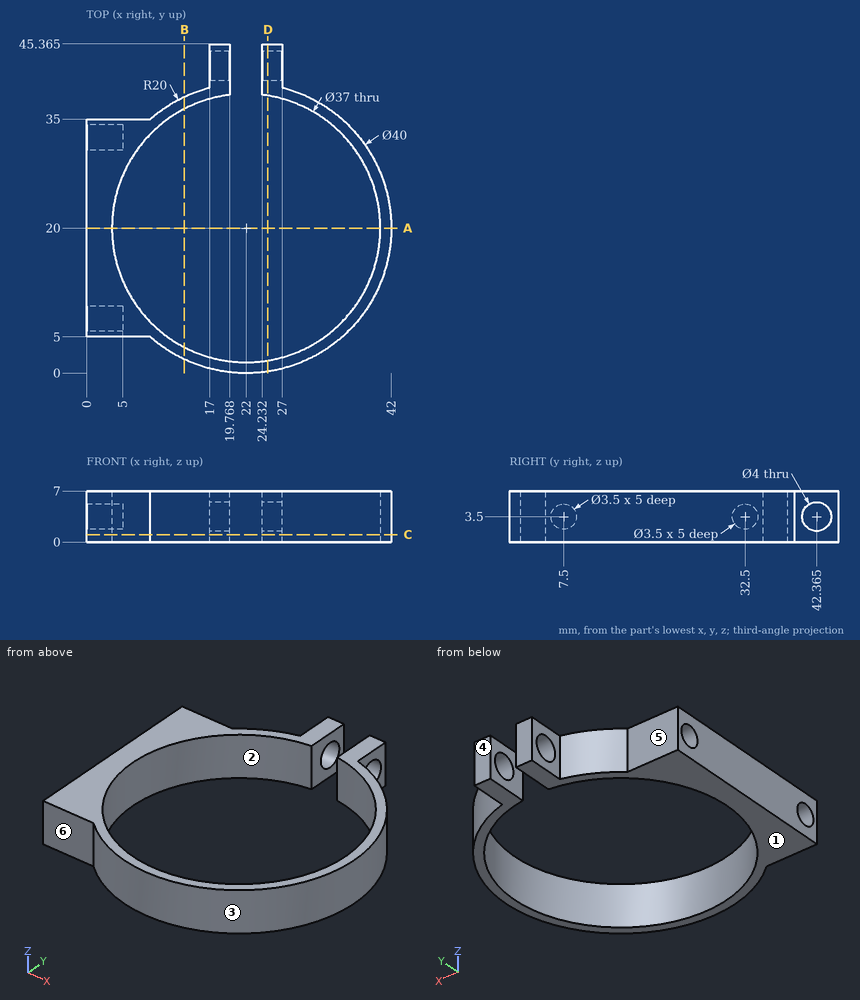
Geometry check sheet. Reference: drawing and pictorial views, mm from the part's lowest x, y, z. A direction names the side the tool comes from. Coordinates: 2 decimals unless noted, no trailing zeros. Order: outer loops, then holes, each group sorted by start corner. A loop starts at its lowest first (then second) coordinate and runs counter-clockwise, first axis right, second up.
Item 1: Mould release check, pull along X, two halves, no side actions. Record for the marked faces 1, 2 and 3: released by +X, released by -X, zero draft, split by the parting line, or undercut.
Item 2: Scan lines: line 1 along Y through (x, z) = (2, 3.5); line 2 along Y through (x, z) = (26, 2) (1 decimal); line 3 along Z through (x, y) = (2, 32.5). Record each from-to range of solid material in increasing order.
Item 3: Section check B-B (x = 13.5). Enter the section's corners in (y, z), plus the area to 3 significant figures.
Item 4: Tool access check on the marked faces 4, 5 and 6. Record the directions out of +Z, -Z, +X, -X, +Y, -Y that give a thin tool (end or side, any length) a straight path to the whole face; none if there is none.
Item 5: Depth check by flat-ended pin: pin 1 (3 mm diameter, centred on y = 43.5, z = 3.5, fed in from -X); pin 2 (2 mm diameter, centred on y = 26.5, z = 4.5, fed in from -X); pin 3 (1.8 mm diameter, centred on y = 32, z = 3.5, fed in from -X); pin 4 (2 mm diameter, centred on y = 40.5, z = 4, fed in from +X). Enter the tip coordinate at first touch or a pass-through.
Item 6: Section check C-C (z = 1). Enter the section's corners in (x, y) (1 decimal).
Item 7: Section check A-A (y = 20). Enter the section's corners in (x, z), plus the area to 3 significant figures.
Item 8: Section check D-D (x = 25). Enter the section's corners in (y, z) (1 decimal).
Check sheet entries:
1. face 1: zero draft
1. face 2: undercut
1. face 3: split by the parting line
2. line 1: y = 5 to 5.75, 9.25 to 30.75, 34.25 to 35
2. line 2: y = 0.4 to 1.9, 38.1 to 41, 43.7 to 45.4
2. line 3: z = 0 to 1.75, 5.25 to 7
3. outline: (1.9, 0) - (3.57, 0) - (3.57, 7) - (1.9, 7) - close; (36.43, 0) - (38.1, 0) - (38.1, 7) - (36.43, 7) - close
3. area: 23.4 mm2
4. face 4: +Z, -Z, +X, -X, +Y
4. face 5: +Z, -Z, -X, +Y
4. face 6: +Z, -Z, -X, -Y
5. pin 1: stops at x = 17
5. pin 2: stops at x = 0
5. pin 3: stops at x = 5
5. pin 4: stops at x = 27
6. outline: (0, 5) - (8.8, 5) arc R20 ccw (long way) to (27, 39.4) - (27, 45.4) - (24.2, 45.4) - (24.2, 38.4) arc R18.5 cw (long way) to (19.8, 38.4) - (19.8, 45.4) - (17, 45.4) - (17, 39.4) arc R20 ccw to (8.8, 35) - (0, 35) - close
7. outline: (0, 0) - (3.5, 0) - (3.5, 7) - (0, 7) - close; (40.5, 0) - (42, 0) - (42, 7) - (40.5, 7) - close
7. area: 35.0 mm2
8. outline: (0.2, 0) - (1.7, 0) - (1.7, 7) - (0.2, 7) - close; (38.3, 0) - (45.4, 0) - (45.4, 7) - (38.3, 7) - close; hole circle Ø4 at (42.4, 3.5)
